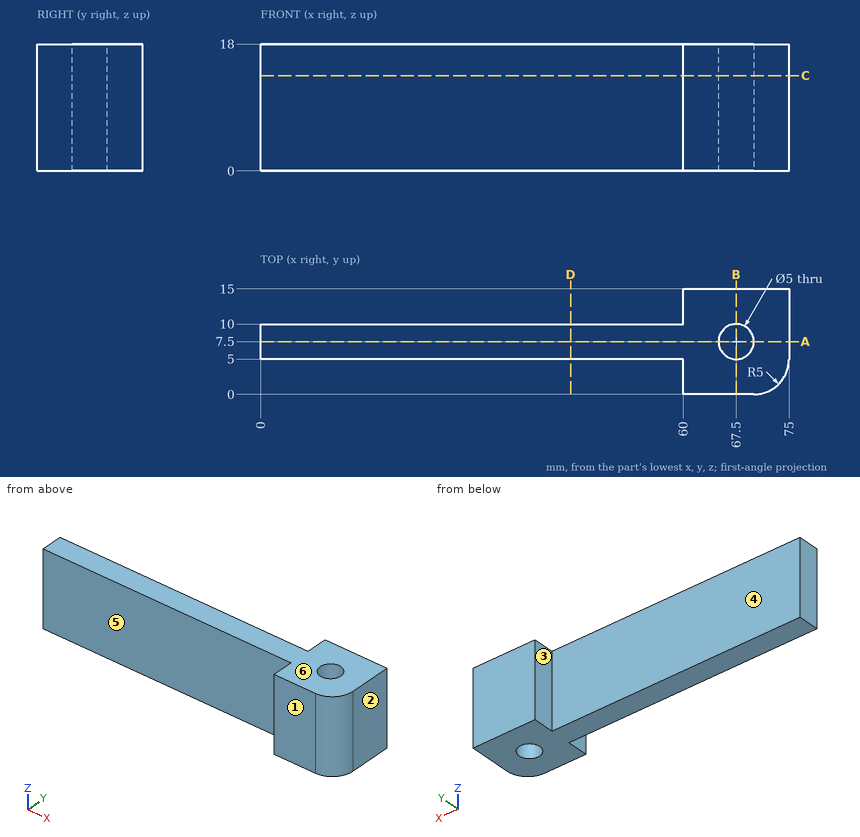
Input: dimensioned drawing with shaded views. Units: mm. Origin: part minimum x, y, z. A direction names the side the tool comes from. Round coordinates to 2 decimals unless told otherwise and drop trailing zeros. Write each loop counter-clockwise with the first axis right and the second up, starting at its lowest first coordinate (ties: lowest second). Pieces come first, ordered by that corner, then holes. Notation, with made-up numbers: (49, 61) - (98, 61) arc R11 cw to (98, 78) - close; hole circle Ø3 at (70, 50). An arc over 180 degrees is marked (long way). Write item = value, one per line.
(1) Contact query for flat-ended pins moving along their axis: pin 1 Ø6 at (x, z) = (40, 10.5) entering from +Y; pin 2 Ø2 at (x, z) = (57, 6) entering from -Y; pin 3 Ø1.5 at (y, z) = (12.5, 8) entering from -X. Output: stop coordinate, or through.
Geometry check:
pin_1 = 10
pin_2 = 5
pin_3 = 60
(2) Section query D-D on x = 44. Output: boundary loops of the cut face in (y, z), then the cut area to 3 significant figures.
Geometry check:
outline = (5, 0) - (10, 0) - (10, 18) - (5, 18) - close
area = 90.0 mm^2
(3) Section query B-B on x = 67.5. Output: boundary loops of the cut face in (y, z), then the cut area to 3 significant figures.
Geometry check:
outline = (0, 0) - (5, 0) - (5, 18) - (0, 18) - close; (10, 0) - (15, 0) - (15, 18) - (10, 18) - close
area = 180 mm^2
(4) Section query C-C on z = 13.5. Output: boundary loops of the cut face in (x, y).
Geometry check:
outline = (0, 5) - (60, 5) - (60, 0) - (70, 0) arc R5 ccw to (75, 5) - (75, 15) - (60, 15) - (60, 10) - (0, 10) - close; hole circle Ø5 at (67.5, 7.5)
(5) Section query A-A on y = 7.5. Output: boundary loops of the cut face in (x, z), then the cut area to 3 significant figures.
Geometry check:
outline = (0, 0) - (65, 0) - (65, 18) - (0, 18) - close; (70, 0) - (75, 0) - (75, 18) - (70, 18) - close
area = 1,260 mm^2
(6) Access query for the marked faces 4, 5 and 6. Directions: +Z, -Z, +X, -X, +Y, -Y. A direction counts if a zero-diameter tool reaches every point of the face in a straight line with its end or side. Return the directions, or none.
Geometry check:
face_4 = +Z, -Z, -X, +Y
face_5 = +Z, -Z, -X, -Y
face_6 = +Z, +X, -X, +Y, -Y
(7) Pull-direction query (X, two-part tool) for the marked faces 1, 2 and 3; classes: +X half, -X half, draft (parallel to the pull), parting line (faces both ways), or undercut.
Geometry check:
face_1 = draft
face_2 = +X half
face_3 = -X half
(8) Material intervals for probe 1 along X at (y, z) = (7.75, 14.5); probe 2 along Y at (x, z) = (67.5, 10.5); probe 3 along X at (y, z) = (11.5, 6.5), sorted ascending.
Geometry check:
probe_1 = 0 to 65.01, 69.99 to 75
probe_2 = 0 to 5, 10 to 15
probe_3 = 60 to 75
